Answer from the drawing. Dimensions are ordinates in mm from the lowest x, y and z of the part. A direction names the side the tool comes from. Round coordinates to 2 decimals unless told otherwise and drop trailing zeros. Loops run counter-clockwise (first coordinate to the right, second up) from the corner with the lowest first, then second, coordinate; pieces in that order, holes last. Notation, with made-up numbers: M 15,45.25 L 44,45.25 A19 cw 44,62.25 Z; hole C 58,-24 d2. An arc over 180 degrees is marked long. One line per item, written item: value.
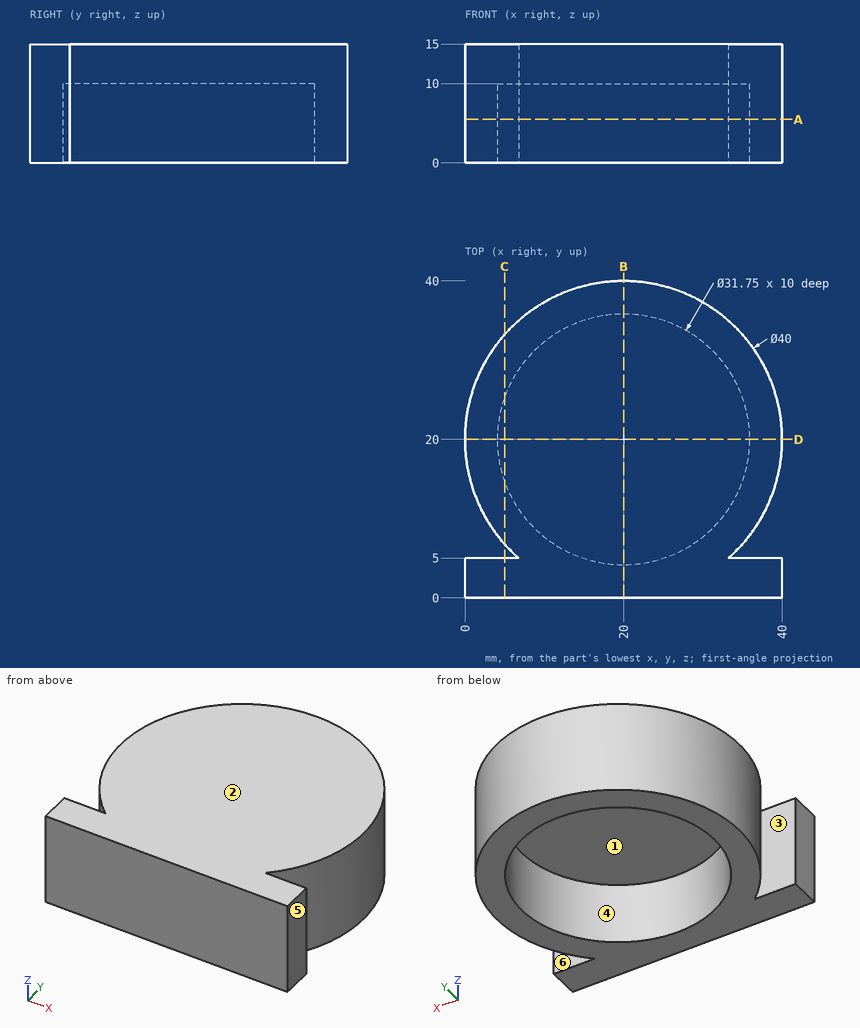
1) Each of these flat-tipped pins is pushed along its axis until it touches: pin 1 (2 mm diameter, centred on y = 24, z = 11.5, fed in from -X); pin 2 (1 mm diameter, centred on y = 18.5, z = 6.5, fed in from -X) (3 decimals); pin 3 (1.5 mm diameter, centred on x = 35.5, z = 3, fed in from +Y). Where does it stop, or does it pass through?
Check values:
pin 1: x = 0.23
pin 2: x = 0.025
pin 3: y = 33.51
2) Find section B-B (x = 20). Give the vertices of the cut face in (y, z) (3 decimals), then the cut area to 4 significant figures.
Check values:
outline: M 0,0 L 4.125,0 L 4.125,10 L 35.875,10 L 35.875,0 L 40,0 L 40,15 L 0,15 Z
area: 282.5 mm2
3) For the marked faces 1, 2 and 3, determine the directions among +Z, -Z, +X, -X, +Y, -Y from which every point of the face is accessible in a straight line to the end or side of a thin tool.
Check values:
face 1: -Z
face 2: +Z, +X, -X, +Y, -Y
face 3: +Z, -Z, -X
4) Find section A-A (z = 5.5). Give the vertices of the cut face in (x, y) (3 decimals), then the cut area to 3 significant figures.
Check values:
outline: M 0,0 L 40,0 L 40,5 L 33.229,5 A20 ccw long 6.771,5 L 0,5 Z; hole C 20,20 d31.75
area: 574 mm2
5) Find the intervals of material crossed by probe 1 along Y at (x, z) = (20, 2.5) (3 decimals); probe 2 along Z at (x, y) = (9, 21); probe 3 along Y at (x, z) = (15, 9.25), in increasing order. Write a range as from..to.
Check values:
probe 1: 0..4.125, 35.875..40
probe 2: 10..15
probe 3: 0..4.93, 35.07..39.36
6) Find section C-C (x = 5). Give the vertices of the cut face in (y, z).
Check values:
outline: M 0,0 L 5,0 L 5,15 L 0,15 Z; M 6.77,0 L 14.8,0 L 14.8,10 L 25.2,10 L 25.2,0 L 33.23,0 L 33.23,15 L 6.77,15 Z
7) The mould has two halves that part along X. Classify the marked faces 4, 5 and 6: +X half, -X half, draft (parallel to the pull), parting line (faces both ways), or undercut.
Check values:
face 4: undercut
face 5: +X half
face 6: draft
